from build123d import *

# Parameters (mm, degrees)
SKETCH015_R             = 2.5
SKETCH015_R_2           = 11
SKETCH015_R_3           = 1.5
PAD_DEPTH               = 6.35
BODY004_PLACEMENT_ANGLE = 0.285111


with BuildPart() as part:
    # Sketch015 → Pad (new body)
    with BuildSketch(Plane(origin=(0, 0, 0), x_dir=(1, 0, 0), z_dir=(0, 0, -1))):
        Polygon((-60, -6.5), (-60, 94.5), (-55, 99.5), (-45, 99.5), (-40, 94.5), (-40, 36.5), (-35, 31.5), (35, 31.5), (40, 36.5), (40, 94.5), (45, 99.5), (55, 99.5), (60, 94.5), (60, -35.175), (64.825, -40), (64.825, -95), (59.825, -100), (49.825, -100), (44.825, -95), (44.825, -40.175), (39.825, -35.175), (-4.715729, -35.175), (-44.825, -75.284271), (-44.825, -122), (-49.825, -127), (-59.825, -127), (-64.825, -122), (-64.825, -67), (-35.698034, -37.873034), (-35.698034, -30.801966), align=None)
        with Locations((-50, 89.5)):
            Circle(SKETCH015_R, mode=Mode.SUBTRACT)
        with Locations((-50, 36.5)):
            Circle(SKETCH015_R, mode=Mode.SUBTRACT)
        with Locations((50, 36.5)):
            Circle(SKETCH015_R, mode=Mode.SUBTRACT)
        Circle(SKETCH015_R_2, mode=Mode.SUBTRACT)
        with Locations((50, 89.5)):
            Circle(SKETCH015_R, mode=Mode.SUBTRACT)
        with Locations((-12.5, 12.5)):
            Circle(SKETCH015_R_3, mode=Mode.SUBTRACT)
        with Locations((12.5, 12.5)):
            Circle(SKETCH015_R_3, mode=Mode.SUBTRACT)
        with Locations((12.5, -12.5)):
            Circle(SKETCH015_R_3, mode=Mode.SUBTRACT)
        with Locations((-12.5, -12.5)):
            Circle(SKETCH015_R_3, mode=Mode.SUBTRACT)
        with Locations((-50, 3.5)):
            Circle(SKETCH015_R, mode=Mode.SUBTRACT)
        with Locations((-50, 56.5)):
            Circle(SKETCH015_R, mode=Mode.SUBTRACT)
        with Locations((50, 56.5)):
            Circle(SKETCH015_R, mode=Mode.SUBTRACT)
        with Locations((50, 3.5)):
            Circle(SKETCH015_R, mode=Mode.SUBTRACT)
        with BuildLine():
            ThreePointArc((-53.275, -77), (-54.825, -75.45), (-56.375, -77))
            Line((-56.375, -77), (-56.375, -117))
            ThreePointArc((-56.375, -117), (-54.825, -118.55), (-53.275, -117))
            Line((-53.275, -117), (-53.275, -77))
        make_face(mode=Mode.SUBTRACT)
        with BuildLine():
            ThreePointArc((56.375, -50), (54.825, -48.45), (53.275, -50))
            Line((53.275, -50), (53.275, -90))
            ThreePointArc((53.275, -90), (54.825, -91.55), (56.375, -90))
            Line((56.375, -90), (56.375, -50))
        make_face(mode=Mode.SUBTRACT)
    extrude(amount=PAD_DEPTH)


with BuildPart() as part_1:
    # Body004 placement: moved
    add(part.part.moved(Location((45.071194, -32.948698, 1.778014))).rotate(Axis((45.071194, -32.948698, 1.778014), (0, 0, 1)), BODY004_PLACEMENT_ANGLE))


solid = part_1.part
Input: part model. Units: mm. Frame: model coordinates. Give positions to 0.01 mm unless a question says otherwise; leave off trailing zeros. Order: outer loops, then holes, each group sorted by start corner. A loop starts at its lowest first (then second) coordinate and runs counter-clockwise, first axis right, second up.
Q1. Contact query for flat-ended pins moving along their axis: pin 1 Ø1 at (y, z) = (-88, -4) entering from +X; pin 2 Ø1.5 at (y, z) = (-64.5, -3) entering from +X; pin 3 Ø1.5 at (y, z) = (-84.5, 1) entering from -X. Output: stop coordinate, or through.
Checked values:
pin 1: stops at x = 105.35
pin 2: stops at x = 105.23
pin 3: stops at x = -14.68
Q2. Draft query along X for faces 1 (the flat face through (107.26, 4.91, -1.35)), 2 (the flat face through (-2.701, -14.365, -1.353)), 3 (the flat face through (20.308, 21.878, -1.353)). Return one class per face: +X half, -X half, draft (parallel to the pull), parting line (faces both ways), or undercut.
Checked values:
face 1: +X half
face 2: -X half
face 3: undercut
Q3. Section B-B on x = 36.5. Output: boundary loops of the cut face in (y, z).
Checked values:
outline: (-64.49, -4.57) - (-39.84, -4.57) - (-39.84, 1.78) - (-64.49, 1.78) - close; (-26.05, -4.57) - (5.85, -4.57) - (5.85, 1.78) - (-26.05, 1.78) - close
Q4. Section C-C on y = -74.5. Output: boundary loops of the cut face in (x, z), and give its area (3 significant figures).
Checked values:
outline: (-14.72, -4.57) - (5.28, -4.57) - (5.28, 1.78) - (-14.72, 1.78) - close; (85.28, -4.57) - (105.28, -4.57) - (105.28, 1.78) - (85.28, 1.78) - close
area: 254 mm2
Q5. Section A-A on y = 48. Output: boundary loops of the cut face in (x, z).
Checked values:
outline: (-20.16, -4.57) - (-11.71, -4.57) - (-11.71, 1.78) - (-20.16, 1.78) - close; (-8.61, -4.57) - (-0.16, -4.57) - (-0.16, 1.78) - (-8.61, 1.78) - close; (89.49, -4.57) - (97.94, -4.57) - (97.94, 1.78) - (89.49, 1.78) - close; (101.04, -4.57) - (109.49, -4.57) - (109.49, 1.78) - (101.04, 1.78) - close
Q6. Ray query, probe 1 along X at (y, z) = (41.5, 0.75); probe 2 along X at (y, z) = (-20, 0.25); probe 3 along X at (y, z) = (81, 0.75). Return the intervals inside material, ascending.
Checked values:
probe 1: x = -20.13 to 0.49, 89.53 to 97.98, 101.08 to 109.53
probe 2: x = -8.28 to 31.1, 33.92 to 56.06, 58.96 to 105.01
probe 3: x = -20.32 to -11.87, -8.77 to -0.32
Q7. Section D-D on z = -2. State how many separate pieces and enclosed holes the cut face has, and give its area (3 significant figures).
Checked values:
separate pieces: 1
enclosed holes: 15
area: 12,900 mm2
